The figure shows three views and two pictorial views of one solid part (mm, origin at its lowest corner). Answer the questions. Give positions to 0.01 mm unless a question says otherwise; leave off trailing zeros. Order: outer loops, then holes, each group sorted by start corner. A loop starts at its lowest first (then second) coordinate and runs counter-clockwise, first axis right, second up. Notation, with made-up numbers: (-31.75, -34.75) -> (-13.75, -34.75) arc R13 ccw to (-13.75, -23.75) -> close; hole circle Ø3 at (73, 87). An arc over 180 degrees is marked (long way). Use one line per item in the form item = value.
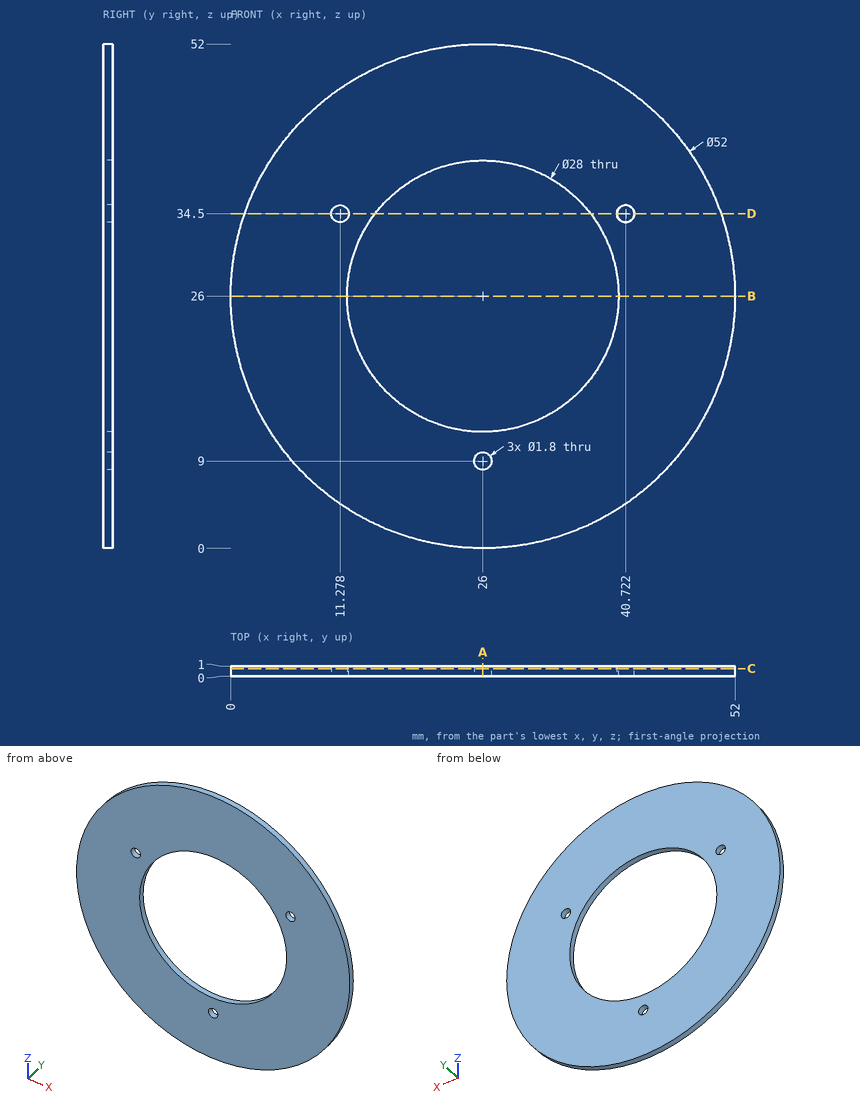
Item 1: Given pin 1 Ø1.6 at (x, z) = (11.28, 34.5) entering from +Y, flat-ended and moving along its own axis, determine where the tip first touches the part or whether it passes through.
Checks:
pin_1 = through
Item 2: The part is cut by section A-A on x = 26. Give the vertices of the cut face in (y, z), and give its area (3 significant figures).
Checks:
outline = (0, 0) -> (1, 0) -> (1, 8.1) -> (0, 8.1) -> close; (0, 9.9) -> (1, 9.9) -> (1, 12) -> (0, 12) -> close; (0, 40) -> (1, 40) -> (1, 52) -> (0, 52) -> close
area = 22.2 mm²
Item 3: The part is cut by section B-B on z = 26. Give the vertices of the cut face in (x, y).
Checks:
outline = (0, 0) -> (12, 0) -> (12, 1) -> (0, 1) -> close; (40, 0) -> (52, 0) -> (52, 1) -> (40, 1) -> close
Item 4: The part is cut by section D-D on z = 34.5. Give the vertices of the cut face in (x, y) (1 decimal).
Checks:
outline = (1.4, 0) -> (10.4, 0) -> (10.4, 1) -> (1.4, 1) -> close; (12.2, 0) -> (14.9, 0) -> (14.9, 1) -> (12.2, 1) -> close; (37.1, 0) -> (39.8, 0) -> (39.8, 1) -> (37.1, 1) -> close; (41.6, 0) -> (50.6, 0) -> (50.6, 1) -> (41.6, 1) -> close
Item 5: The part is cut by section C-C on y = 0.75. Give the vertices of the cut face in (x, z), and give its area (3 significant figures).
Checks:
outline = circle Ø52 at (26, 26); hole circle Ø1.8 at (11.28, 34.5); hole circle Ø28 at (26, 26); hole circle Ø1.8 at (26, 9); hole circle Ø1.8 at (40.72, 34.5)
area = 1,500 mm²
Item 6: Straight lines are drawn through the part: L1, parallel to Z at x = 26, y = 0.6; L2, parallel to X at y = 0.45, z = 26; L3, parallel to X at y = 0.35, z = 34.5 (1 decimal). For each, find the intervals that lie inside material, in ascending order. Write a range as from..to.
Checks:
L1 = 0..8.1, 9.9..12, 40..52
L2 = 0..12, 40..52
L3 = 1.4..10.4, 12.2..14.9, 37.1..39.8, 41.6..50.6
